Input: part model. Units: mm. Frame: model coordinates. Face numbers are marked on the shaded views. A direction names the side the tool comes from. Round coordinates to 2 decimals unless told otherwise and drop trailing zeros. Order: outer loops, then holes, each group sorted by start corner. A loop starts at its lowest first (then second) coordinate and runs counter-clockwise, first axis right, second up. Notation, with made-up numbers: (78, 81.25) -> (105, 81.25) arc R16 cw to (105, 111.25) -> close; hole circle Ø3 at (-32.75, 21.25). An arc over 180 degrees is marked (long way). Use a Markdown table: item, result.
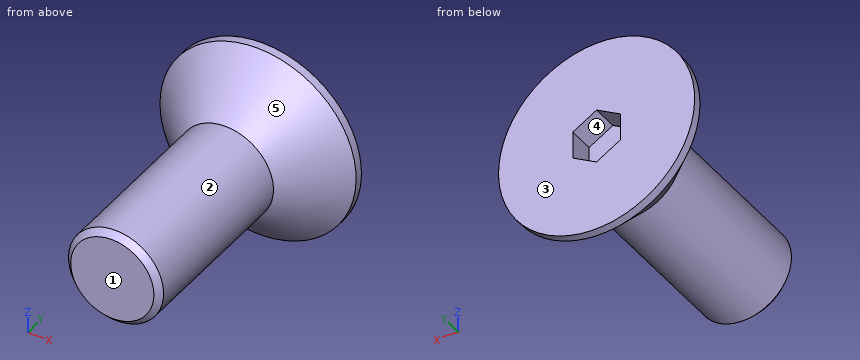
from build123d import *

# Parameters (mm, degrees)
CUT_EXTRUDE1_DEPTH = 2.16
CHAMFER1_SIZE      = 0.5


with BuildPart() as part:
    # Sketch2 → Revolve1 (revolve)
    with BuildSketch(Plane.XY, mode=Mode.PRIVATE) as revolve1_sk:
        Polygon((0, 0), (8.25, 0), (8.25, -0.71), (4, -4.96), (4, -20), (0, -20), align=None)
    revolve(revolve1_sk.sketch.rotate(Axis((0, 0, 0), (0, -1, 0)), 90), axis=Axis((0, 0, 0), (0, -1, 0)))

    # Sketch3 → Cut-Extrude1 (cut)
    with BuildSketch(Plane(origin=(0, 0, 0), x_dir=(1, 0, 0), z_dir=(0, 1, 0))):
        Polygon((0, 2.309401077), (2, 1.154700538), (2, -1.154700538), (0, -2.309401077), (-2, -1.154700538), (-2, 1.154700538), align=None)
    extrude(amount=-CUT_EXTRUDE1_DEPTH, mode=Mode.SUBTRACT)

    # Chamfer1
    chamfer1_edges = [part.edges().sort_by_distance(p)[0] for p in [
        (0, -20, -4),
    ]]
    chamfer(chamfer1_edges, length=CHAMFER1_SIZE)


solid = part.part
1) Cut plane A-A on z = 0. Return loops of the section in (x, y).
Answer key:
| item | result |
|---|---|
| outline | (-8.25, -0.71) -> (-4, -4.96) -> (-4, -19.5) -> (-3.5, -20) -> (3.5, -20) -> (4, -19.5) -> (4, -4.96) -> (8.25, -0.71) -> (8.25, 0) -> (2, 0) -> (2, -2.16) -> (-2, -2.16) -> (-2, 0) -> (-8.25, 0) -> close |
2) Ray query, probe 1 along Y at (x, z) = (2.75, -2.5); probe 2 along Y at (x, z) = (-5.25, -6); probe 3 along Z at (x, y) = (3.25, -1.5). Return the intervals inside material, ascending.
Answer key:
| item | result |
|---|---|
| probe 1 | y = -19.78 to 0 |
| probe 2 | y = -0.99 to 0 |
| probe 3 | z = -6.71 to 6.71 |
3) Cut plane B-B on y = -7.5. Return loops of the section in (x, z).
Answer key:
| item | result |
|---|---|
| outline | circle Ø8 at (0, 0) |
4) Contact query for flat-ended pins moving along their axis: P1, Ø2, axis at x = 0, z = 0.5, coming from the +Y side; P2, Ø1, axis at x = -6.5, z = 5.5, coming from the -Y side; P3, Ø1.1, axis at y = -1.5, z = 0, coming from the -X side. Output: stop coordinate, or through.
Answer key:
| item | result |
|---|---|
| P1 | stops at y = -2.16 |
| P2 | stops at y = -0.95 |
| P3 | stops at x = -8.01 |
5) Set-up query: the marked faces 1 and 2. Return all of +Z, -Z, +X, -X, +Y, -Y with unobstructed straight access to the full face (end or side cutting, diameter ignored); none if empty.
Answer key:
| item | result |
|---|---|
| face 1 | +Z, -Z, +X, -X, -Y |
| face 2 | -Y |
6) Draft query along Z for the marked faces 3, 4 and 5. Return one class per face: released by +Z, released by -Z, zero draft, split by the parting line, or undercut.
Answer key:
| item | result |
|---|---|
| face 3 | zero draft |
| face 4 | undercut |
| face 5 | split by the parting line |
